Can you work these out from the model? Positions are in its coordinate system, mm. A direction names the side the tool comes from. Round coordinates to 2 decimals unless told otherwise and drop trailing zeros. Loops run counter-clockwise (first coordinate to the right, second up) from the corner with the lowest first, then second, coordinate; pieces in that order, holes last.
(1) Which directions (+Z, -Z, +X, -X, +Y, -Y) give clear straight access to the entire face, cutting with the end or side of a thin tool? Please do faces 5 (the face through (0.36, -0.99, 3.15)), 6 (the face through (-26.652, -7.555, -0.992)).
(2) I want a section at C-C on z = 6.5. Write out the boundary of the cut face in (x, y), plus the area to 3 significant figures.
(3) If I drill on line 1 along X through (y, z) = (-4.75, -1.75); line 2 along Z through (x, y) = (-22.5, -0.5); line 3 along Z through (x, y) = (23.5, 2.25), over which ranges is the centre line in solid material (lowest first)?
(4) Will these pins go through, and if not, where does the flat tip stop? pin 1 Ø1 at (x, y) = (35.5, 4.5) entering from +Z; pin 2 Ø1.5 at (x, z) = (-7.5, 0.5) entering from +Y; pin 3 Ø6 at (x, z) = (38, 6) entering from -Y; pin 4 Ø4 at (x, z) = (2, 3) entering from +Y.
(5) I want a section at D-D on x = 34.5. Write out the boundary of the cut face in (y, z), plus the area to 3 significant figures.
(6) I want a section at A-A on y = 0. Write out the boundary of the cut face in (x, z), plus the area to 3 significant figures.
(7) Thinking about a two-plate mould opening in X: for faces 1 (the face through (-55.88, 0, 0)), 2 (the face through (27.94, 2, -3)), 3 (the face through (-53.34, 2, -3)), 4 (the face through (-54.592, -7.555, -0.992)), which applies, released by +X, released by -X, zero draft, split by the parting line, or undercut?
from build123d import *

# Parameters (mm, degrees)
SKETCH1_W = 111.76
SKETCH1_H = 3.302
SKETCH6_W = 2.54
SKETCH6_H = 4.318


with BuildPart() as part:
    # Sketch1 → Revolve1 (revolve)
    with BuildSketch(Plane.XY, mode=Mode.PRIVATE) as revolve1_sk:
        with Locations((0, 1.651)):
            Rectangle(SKETCH1_W, SKETCH1_H)
    revolve(revolve1_sk.sketch.rotate(Axis((-55.88, 0, 0), (1, 0, 0)), 90), axis=Axis((-55.88, 0, 0), (1, 0, 0)))

    # Sketch6 → Revolve2 (revolve)
    with BuildSketch(Plane.XY, mode=Mode.PRIVATE) as revolve2_sk:
        with Locations((-26.67, 5.461)):
            Rectangle(SKETCH6_W, SKETCH6_H)
        with Locations((26.67, 5.461)):
            Rectangle(SKETCH6_W, SKETCH6_H)
        with Locations((-54.61, 5.461)):
            Rectangle(SKETCH6_W, SKETCH6_H)
        with Locations((54.61, 5.461)):
            Rectangle(SKETCH6_W, SKETCH6_H)
    revolve(revolve2_sk.sketch.rotate(Axis((-31.878421892, 0, 0), (1, 0, 0)), 90), axis=Axis((-31.878421892, 0, 0), (1, 0, 0)))


solid = part.part
Filled sheet:
1. face 5: none
1. face 6: +X, -X
2. outline: (-55.88, -3.98) - (-53.34, -3.98) - (-53.34, 3.98) - (-55.88, 3.98) - close; (-27.94, -3.98) - (-25.4, -3.98) - (-25.4, 3.98) - (-27.94, 3.98) - close; (25.4, -3.98) - (27.94, -3.98) - (27.94, 3.98) - (25.4, 3.98) - close; (53.34, -3.98) - (55.88, -3.98) - (55.88, 3.98) - (53.34, 3.98) - close
2. area: 80.8 mm2
3. line 1: x = -55.88 to -53.34, -27.94 to -25.4, 25.4 to 27.94, 53.34 to 55.88
3. line 2: z = -3.26 to 3.26
3. line 3: z = -2.42 to 2.42
4. pin 1: passes through
4. pin 2: stops at y = 3.3
4. pin 3: stops at y = -1.38
4. pin 4: stops at y = 3.15
5. outline: circle Ø6.6 at (0, 0)
5. area: 34.3 mm2
6. outline: (-55.88, -7.62) - (-53.34, -7.62) - (-53.34, -3.3) - (-27.94, -3.3) - (-27.94, -7.62) - (-25.4, -7.62) - (-25.4, -3.3) - (25.4, -3.3) - (25.4, -7.62) - (27.94, -7.62) - (27.94, -3.3) - (53.34, -3.3) - (53.34, -7.62) - (55.88, -7.62) - (55.88, 7.62) - (53.34, 7.62) - (53.34, 3.3) - (27.94, 3.3) - (27.94, 7.62) - (25.4, 7.62) - (25.4, 3.3) - (-25.4, 3.3) - (-25.4, 7.62) - (-27.94, 7.62) - (-27.94, 3.3) - (-53.34, 3.3) - (-53.34, 7.62) - (-55.88, 7.62) - close
6. area: 826 mm2
7. face 1: released by -X
7. face 2: undercut
7. face 3: undercut
7. face 4: zero draft
